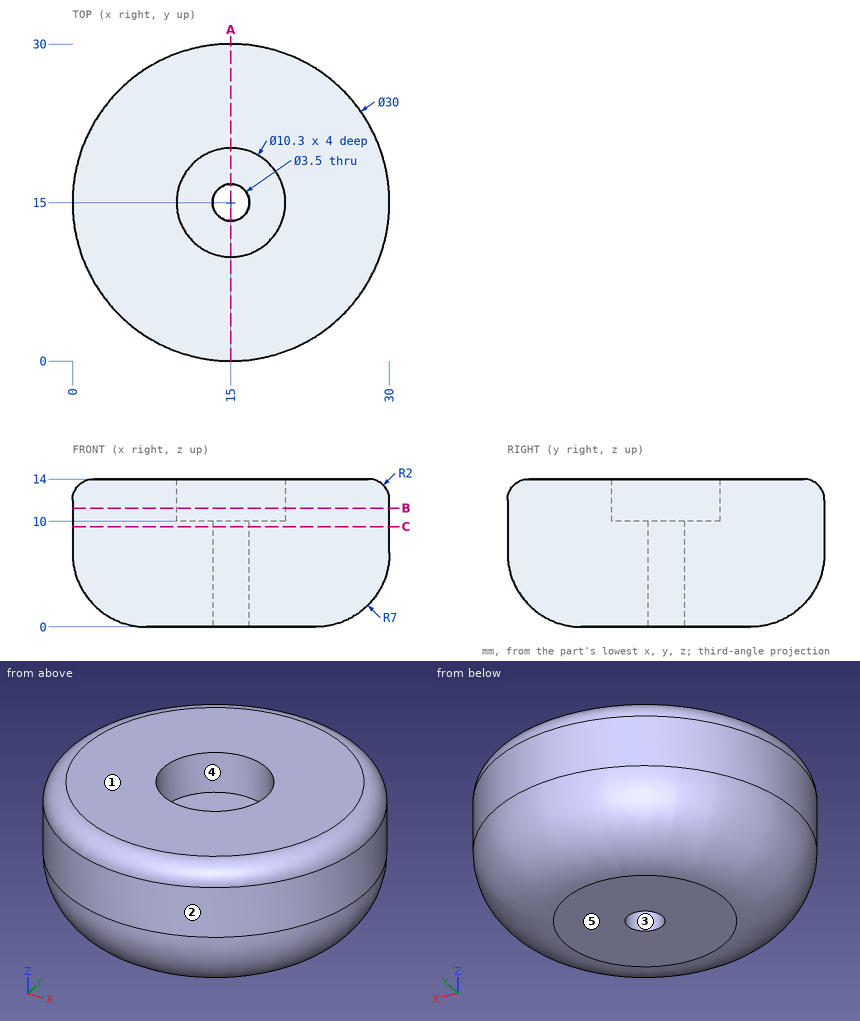
Input: dimensioned drawing with shaded views. Units: mm. Origin: part minimum x, y, z. A direction names the side the tool comes from. Give positions to 0.01 mm unless a question says otherwise; leave off trailing zeros. Order: outer loops, then holes, each group sorted by start corner. A loop starts at its lowest first (then second) coordinate and runs counter-clockwise, first axis right, second up.
(1) Section query B-B (z = 11.25). Return the cut outline in (x, y).
(2) Contact query for flat-ended pins moving along their axis: P1, Ø1.5, axis at x = 25.5, z = 12.5, coming from the +Y side; P2, Ø2, axis at y = 26.5, z = 2.5, coming from the -X side; P3, Ø2, axis at y = 8.5, z = 3.5, coming from the -X side. Output: stop coordinate, or through.
(3) Access query for the marked faces 4 and 5. Directions: +Z, -Z, +X, -X, +Y, -Y. A direction counts if a zero-diameter tool reaches every point of the face in a straight line with its end or side. Return the directions, or none.
(4) Material intervals for line 1 along Y through (x, z) = (15, 8.25); line 2 along Y through (x, z) = (15, 11.85); line 3 along Z through (x, y) = (25, 4.5), sorted ascending.
(5) Pull-direction query (Y, two-part tool) for the marked faces 1, 2 and 3; classes: +Y half, -Y half, draft (parallel to the pull), parting line (faces both ways), or undercut.
(6) Section query C-C (z = 9.5). Return the cut outline in (x, y).
(7) Section query A-A (x = 15). Return the cut outline in (y, z).
Outcome:
1. outline: circle Ø30 at (15, 15); hole circle Ø10.3 at (15, 15)
2. P1: stops at y = 26.35
2. P2: stops at x = 6.26
2. P3: stops at x = 1.8
3. face 4: +Z
3. face 5: -Z, +X, -X, +Y, -Y
4. line 1: y = 0 to 13.25, 16.75 to 30
4. line 2: y = 0 to 9.85, 20.15 to 30
4. line 3: z = 4.4 to 13.32
5. face 1: draft
5. face 2: parting line
5. face 3: undercut
6. outline: circle Ø30 at (15, 15); hole circle Ø3.5 at (15, 15)
7. outline: (0, 7) arc R7 ccw to (7, 0) - (13.25, 0) - (13.25, 10) - (9.85, 10) - (9.85, 14) - (2, 14) arc R2 ccw to (0, 12) - close; (16.75, 0) - (23, 0) arc R7 ccw to (30, 7) - (30, 12) arc R2 ccw to (28, 14) - (20.15, 14) - (20.15, 10) - (16.75, 10) - close
